Source: CAD feature listing. Evaluate the final solid. Frame: model axes, mm. Face numbers are marked on the shaded views. Round coordinates to 2 decimals unless told otherwise and drop trailing zeros. Write each loop counter-clockwise with the first axis right and the second up, starting at its lowest first coordinate (ties: lowest second). Pieces come first, ordered by that corner, then holes. Notation, with made-up numbers: M 31.5,-21.75 L 52.5,-21.75 A20 ccw 52.5,-5.75 Z; hole C -20,53 d10. An arc over 180 degrees is marked long. Answer in a Markdown table with one row per item.
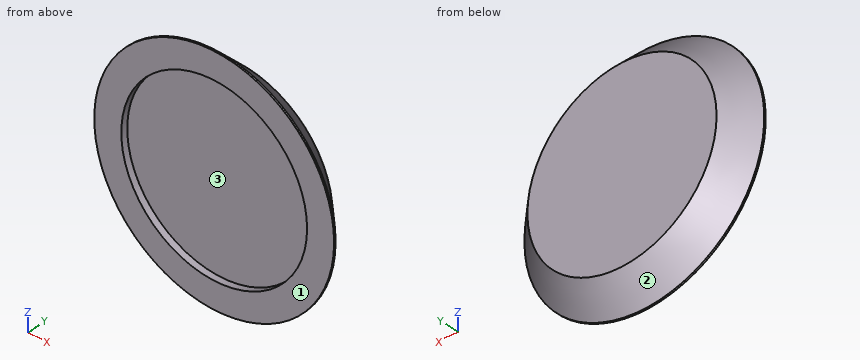
from build123d import *

# Parameters (mm, degrees)
F0_R     = 45.085
F1_DEPTH = 10.16
F2_R     = 34.925
F3_DEPTH = 2.54
F4_SIZE  = 9.525


with BuildPart() as f1:
    # F0 (on Front) → F1 (new body)
    with BuildSketch(Plane.XZ):
        Circle(F0_R)
    extrude(amount=F1_DEPTH)

    # F2 (on face) → F3 (cut)
    with BuildSketch(Plane.XZ.offset(10.16)):
        Circle(F2_R)
    extrude(amount=-F3_DEPTH, mode=Mode.SUBTRACT)

    # F4
    f4_edges = [f1.edges().sort_by_distance(p)[0] for p in [
        (-45.085, 0, 0),
    ]]
    chamfer(f4_edges, length=F4_SIZE)


solid = f1.part
Q1. Material intervals for probe 1 along Z at (x, y) = (0, -9.1) (3 decimals); probe 2 along Y at (x, z) = (28.5, -19); probe 3 along Z at (x, y) = (0, -8.65) (3 decimals), sorted ascending.
Solutions:
| item | result |
|---|---|
| probe 1 | z = -44.66 to -34.925, 34.925 to 44.66 |
| probe 2 | y = -7.62 to 0 |
| probe 3 | z = -44.21 to -34.925, 34.925 to 44.21 |
Q2. Contact query for flat-ended pins moving along their axis: pin 1 Ø1 at (y, z) = (-8.5, 10.5) entering from +X; pin 2 Ø2 at (x, y) = (-20, -6) entering from +Z; pin 3 Ø4 at (x, y) = (-19, -6.5) entering from -Z. Output: stop coordinate, or through.
Solutions:
| item | result |
|---|---|
| pin 1 | stops at x = 43.32 |
| pin 2 | stops at z = 37.68 |
| pin 3 | stops at z = -39.94 |
Q3. Section B-B (y = -3.5). Return loops of the section in (x, z).
Solutions:
| item | result |
|---|---|
| outline | C 0,0 d78.12 |
Q4. Pull-direction query (X, two-part tool) for the marked faces 1, 2 and 3; classes: pulls with the +X half, pulls with the -X half, needs draft (parallel to the pull), parting line crosses it, or undercut.
Solutions:
| item | result |
|---|---|
| face 1 | needs draft |
| face 2 | parting line crosses it |
| face 3 | undercut |
Q5. Section A-A (x = 0). Return loops of the section in (y, z) (3 decimals), and give its area (3 significant figures).
Solutions:
| item | result |
|---|---|
| outline | M -10.16,-45.085 L -9.525,-45.085 L 0,-35.56 L 0,35.56 L -9.525,45.085 L -10.16,45.085 L -10.16,34.925 L -7.62,34.925 L -7.62,-34.925 L -10.16,-34.925 Z |
| area | 648 mm2 |
